Autodesk Inventor part; units mm, degrees
ref_plane "YZ Plane" through (0, 0, 0) normal (1, 0, 0) x (0, 1, 0)
ref_plane "XZ Plane" through (0, 0, 0) normal (0, 1, 0) x (-1, 0, 0)
ref_plane "XY Plane" through (0, 0, 0) normal (0, 0, 1) x (1, 0, 0)
sketch "スケッチ1" plane through (0, 0, 0) normal (1, 0, 0) x (0, 1, 0)
  line L0 (0, -0.4) -> (0, 2.4) construction
  line L1 (1.5, 2) -> (2.25, 2)
  line L2 (2.25, 2) -> (2.25, 0.5)
  line L3 (2.25, 0.5) -> (1.5, 0.5)
  line L4 (1.5, 0.5) -> (1.5, 2)
  line L5 (1.5, 0.5) -> (3.75, 0.5)
  line L6 (3.75, 0.5) -> (3.75, 0)
  line L7 (3.75, 0) -> (1.5, 0)
  line L8 (1.5, 0) -> (1.5, 0.5)
  point P0 (0, 0)
  point P1 (2.25, 0.5)
  dimension "d0" = 3
  dimension "d1" = 4.5
  dimension "d2" = 0.5
  dimension "d3" = 2
  dimension "d4" = 7.5
revolve "回転1" add sketch "スケッチ1" angle 360 about axis through (0, 0, -10) along (0, 0, 1)
fillet "フィレット1" radius 0.5 1 edges at (0, -2.25, 0.5)
chamfer "面取り1" distance 0.3 angle 30 1 edges at (0, -2.25, 2) measured on face at (0.181, 2.2427, 1.3333)
properties part number "_GFM-0608-04" material "アセタール樹脂、黒"
Input: part model. Units: mm. Frame: model coordinates. A direction names the side the tool comes from. Round coordinates to 2 decimals unless told otherwise and drop trailing zeros. Loops run counter-clockwise (first coordinate to the right, second up) from the corner with the lowest first, then second, coordinate; pieces in that order, holes last. Notation, with made-up numbers: M 58,28 L 83,28 A10 ccw 83,43 Z; hole C -24.5,67 d11. An arc over 180 degrees is marked long. Answer as CSV lines item,"result". Start each with the question number.
(1) Line query: line 1 (Y direction, x = 0, z = 1.1). Output: solid intervals per line, ascending. Write a range as [from, to].
(2) Reachability of faces 1 (the cylindrical face through (2.23, -0.29, 1.35)), 2 (the flat face through (2, 0, 0)) from +Z, -Z, +X, -X, +Y, -Y: full face, straight path, thin tool, end or side. Return the list, or none.
(3) Section C-C, the plane z = 0.75. Output: boundary loops of the cut face in (x, y), plus the area to 3 significant figures.
(4) Section A-A, the plane y = 0. Output: boundary loops of the cut face in (x, z), plus the area to 3 significant figures.
(5) First-contact query: pin 1 (4 mm diameter, centred on x = 0, y = 0, fed in from -Z). Flat tip, straight axial feed; report the tip coordinate or a pass-through.
Values found:
1,line 1,"y = [-2.25, -1.5], [1.5, 2.25]"
2,face 1,"+Z"
2,face 2,"-Z, +X, -X, +Y, -Y"
3,outline,"C 0,0 d4.63; hole C 0,0 d3"
3,area,"9.80 mm²"
4,outline,"M -3.75,0 L -1.5,0 L -1.5,2 L -2.08,2 L -2.25,1.7 L -2.25,1 A0.5 cw -2.75,0.5 L -3.75,0.5 Z; M 1.5,0 L 3.75,0 L 3.75,0.5 L 2.75,0.5 A0.5 cw 2.25,1 L 2.25,1.7 L 2.08,2 L 1.5,2 Z"
4,area,"4.56 mm²"
5,pin 1,"stops at z = 0"
